Can you work these out from the model? Positions are in its coordinate system, mm. Face numbers are marked on the shaded views. A direction names the side the tool comes from. Coordinates: 2 decimals unless noted, no trailing zeros. Order: outer loops, then holes, each group sorted by start corner. A loop starts at its lowest first (then second) coordinate and runs counter-clockwise, first axis right, second up.
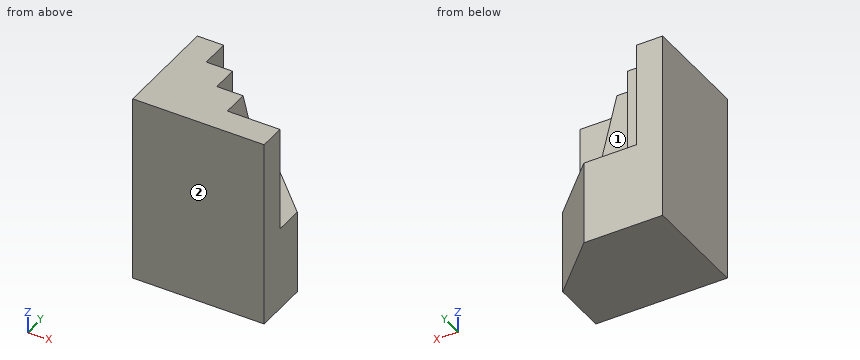
```python
from build123d import *

# Parameters (mm, degrees)
SKETCH1_W           = 1270
SKETCH1_H           = 1828.8
BOSS_EXTRUDE1_DEPTH = 254
BOSS_EXTRUDE2_DEPTH = 812.8
SKETCH3_W           = 254
SKETCH3_H           = 1016
BOSS_EXTRUDE4_DEPTH = 787.4
SKETCH6_W           = 1016
SKETCH6_H           = 508
BOSS_EXTRUDE5_DEPTH = 254
BOSS_EXTRUDE6_DEPTH = 254


with BuildPart() as part:
    # Sketch1 → Boss-Extrude1 (new body)
    with BuildSketch(Plane(origin=(0, 0, 0), x_dir=(1, 0, 0), z_dir=(0, 1, 0))):
        with Locations((635, 914.4)):
            Rectangle(SKETCH1_W, SKETCH1_H)
    extrude(amount=BOSS_EXTRUDE1_DEPTH)

    # Sketch2 → Boss-Extrude2 (add)
    with BuildSketch(Plane(origin=(0, 0, -1828.8), x_dir=(-1, 0, 0), z_dir=(0, 0, -1))):
        Polygon((-1270, 254), (-1270, 533.4), (-762, 1041.4), (0, 1041.4), (0, 254), align=None)
    extrude(amount=-BOSS_EXTRUDE2_DEPTH)

    # Sketch3 → Boss-Extrude4 (add)
    with BuildSketch(Plane(origin=(0, 254, 0), x_dir=(1, 0, 0), z_dir=(0, 1, 0))):
        with Locations((127, 508)):
            Rectangle(SKETCH3_W, SKETCH3_H)
    extrude(amount=BOSS_EXTRUDE4_DEPTH)

    # Sketch6 → Boss-Extrude5 (add)
    with BuildSketch(Plane(origin=(254, 0, 0), x_dir=(0, 0, -1), z_dir=(1, 0, 0))):
        with Locations((508, 508)):
            Rectangle(SKETCH6_W, SKETCH6_H)
    extrude(amount=BOSS_EXTRUDE5_DEPTH)

    # Sketch7 → Boss-Extrude6 (add)
    with BuildSketch(Plane(origin=(0, 254, 0), x_dir=(1, 0, 0), z_dir=(0, 1, 0))):
        Polygon((508, 1016), (1016, 1016), (762, 0), (508, 0), align=None)
    extrude(amount=BOSS_EXTRUDE6_DEPTH)


solid = part.part
```
1. Please list where these lines run through material, in increasing order: probe 1 along Y at (x, z) = (313.5, -995); probe 2 along Z at (x, y) = (1143.5, 362.5); probe 3 along X at (y, z) = (686, -461.5).
Completed:
probe 1: y = 0 to 762
probe 2: z = -1828.8 to -1016
probe 3: x = 0 to 508
2. Imagine slicing it at C-C on y = 835. Please give me the cut outline in (x, z).
Completed:
outline: (0, -1828.8) - (968.4, -1828.8) - (968.4, -1016) - (254, -1016) - (254, 0) - (0, 0) - close
3. I'm going to push flat-ended pins straight in: pin 1 (3 mm diameter, centred on y = 811, z = -821.5, fed in from -X); pin 2 (1.5 mm diameter, centred on x = 919.5, z = -1626, fed in from +Y); pin 3 (3 mm diameter, centred on x = 804, z = -968, fed in from +Y); pin 4 (12 mm diameter, centred on x = 707, y = 630.5, fed in from +Z). Where does each tip first touch, or does it pass through?
Completed:
pin 1: stops at x = 0
pin 2: stops at y = 884.65
pin 3: stops at y = 508
pin 4: stops at z = -1016
4. Imagine slicing it at B-B on x = 1086. Please give me the cut outline in (y, z), then the cut area to 3 significant figures.
Completed:
outline: (0, -1828.8) - (717.4, -1828.8) - (717.4, -1016) - (254, -1016) - (254, 0) - (0, 0) - close
area: 841,000 mm2
5. Imagine slicing it at D-D on x = 883. Please give me the cut outline in (y, z).
Completed:
outline: (0, -1828.8) - (920.4, -1828.8) - (920.4, -1016) - (508, -1016) - (508, -484) - (254, -484) - (254, 0) - (0, 0) - close
6. Imagine slicing it at A-A on z = -180. Please give me the cut outline in (x, y).
Completed:
outline: (0, 0) - (1270, 0) - (1270, 254) - (807, 254) - (807, 508) - (508, 508) - (508, 762) - (254, 762) - (254, 1041.4) - (0, 1041.4) - close
7. On a 3-axis mill with a long thin cutter (end or side, diameter ignored), from which of +Z, -Z, +X, -X, +Y, -Y can I reach the whole of each face in a straight line? I mean the marked faces 1 and 2. Say none if no direction works.
Completed:
face 1: +Z, +X, +Y
face 2: +Z, -Z, +X, -X, -Y
